Source: CAD feature listing. Evaluate the final solid. Frame: model axes, mm. Coordinates: 2 decimals unless noted, no trailing zeros. Order: outer loops, then holes, each group sorted by start corner. A loop starts at its lowest first (then second) coordinate and runs counter-clockwise, first axis right, second up. Notation, with made-up numbers: (36, -2) -> (51, -2) arc R13 cw to (51, 21) -> close; hole circle Ø4 at (56.5, -2). An arc over 180 degrees is marked (long way). Put each result on its own line as item: value.
from build123d import *

# Parameters (mm, degrees)
SKETCH1_W                 = 150
SKETCH1_H                 = 300
BOSS_EXTRUDE1_DEPTH       = 16
SKETCH2_R                 = 5.5
CUT_EXTRUDE4_DEPTH        = 310.646572724
LPATTERN1_COUNT           = 16
LPATTERN1_PITCH           = 16.5
F_8_36_TAPPED_HOLE1_D     = 3.4544
F_8_36_TAPPED_HOLE1_DEPTH = 25
F_8_36_TAPPED_HOLE1_TIP   = 1.037806461


with BuildPart() as part:
    # Sketch1 → Boss-Extrude1 (new body)
    with BuildSketch(Plane.XY):
        with Locations((0, 150)):
            Rectangle(SKETCH1_W, SKETCH1_H)
    extrude(amount=BOSS_EXTRUDE1_DEPTH)

    # Sketch2 → Cut-Extrude4 (cut, through all)
    with BuildSketch(Plane.XY.offset(16)):
        with Locations((60, 37.5)):
            Circle(SKETCH2_R)
    cut_extrude4 = extrude(amount=-CUT_EXTRUDE4_DEPTH, mode=Mode.SUBTRACT)

    # LPattern1: Cut-Extrude4 ×16
    with Locations(*[(0, i * LPATTERN1_PITCH, 0) for i in range(1, LPATTERN1_COUNT)]):
        add(cut_extrude4, mode=Mode.SUBTRACT)

    # #8-36 Tapped Hole1
    with Locations(Plane(origin=(0, 0, 0), x_dir=(-1, 0, 0), z_dir=(0, -1, 0))):
        with Locations((-60, -8), (0, -8), (60, -8)):
            Hole(F_8_36_TAPPED_HOLE1_D / 2, depth=F_8_36_TAPPED_HOLE1_DEPTH)
            with Locations((0, 0, -(F_8_36_TAPPED_HOLE1_DEPTH + F_8_36_TAPPED_HOLE1_TIP / 2))):  # 118° drill point
                Cone(0, F_8_36_TAPPED_HOLE1_D / 2, F_8_36_TAPPED_HOLE1_TIP, mode=Mode.SUBTRACT)


solid = part.part
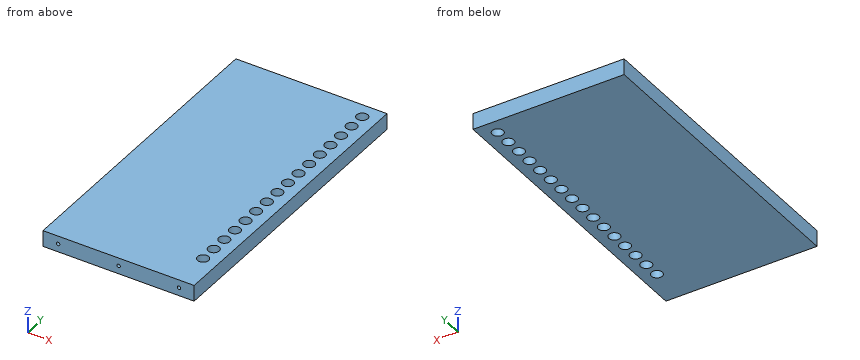
1. Ray query, line 1 along Z through (x, y) = (60, 11.5); line 2 along X through (y, z) = (87.5, 8.5); line 3 along X through (y, z) = (141, 3.25). Return the intervals inside material, ascending.
Numbers:
line 1: z = 0 to 6.27, 9.73 to 16
line 2: x = -75 to 54.52, 65.48 to 75
line 3: x = -75 to 56.84, 63.16 to 75
2. Cut plane A-A on y = 120. Output: boundary loops of the cut face in (x, z), plus the area to 3 significant figures.
Numbers:
outline: (-75, 0) -> (54.5, 0) -> (54.5, 16) -> (-75, 16) -> close; (65.5, 0) -> (75, 0) -> (75, 16) -> (65.5, 16) -> close
area: 2,220 mm2
3. First-contact query: pin 1 (6.5 mm diameter, centred on x = 60, y = 169.5, fed in from -Z). Flat tip, straight axial feed; report the tip coordinate or a pass-through.
Numbers:
pin 1: passes through
